```python
from build123d import *

# Parameters (mm, degrees)
SKETCH1_W           = 207.9625
SKETCH1_H           = 101.6
BOSS_EXTRUDE1_DEPTH = 6.35
SKETCH2_W           = 41.5925
SKETCH2_H           = 6.35
SKETCH2_W_2         = 35.2425
SKETCH2_W_3         = 6.35
SKETCH2_H_2         = 12.7
CUT_EXTRUDE1_DEPTH  = 6.35
SKETCH3_W           = 41.5925
SKETCH3_H           = 31.75
CUT_EXTRUDE2_DEPTH  = 6.35


with BuildPart() as part:
    # Sketch1 → Boss-Extrude1 (new body)
    with BuildSketch(Plane.XY):
        Rectangle(SKETCH1_W, SKETCH1_H)
    extrude(amount=BOSS_EXTRUDE1_DEPTH)

    # Sketch2 → Cut-Extrude1 (cut)
    with BuildSketch(Plane.XY.offset(6.35)):
        with Locations((0, 47.625)):
            Rectangle(SKETCH2_W, SKETCH2_H)
        with Locations((-83.185, 47.625)):
            Rectangle(SKETCH2_W, SKETCH2_H)
        with Locations((83.185, 47.625)):
            Rectangle(SKETCH2_W, SKETCH2_H)
        with Locations((80.01, -47.625)):
            Rectangle(SKETCH2_W_2, SKETCH2_H)
        with Locations((100.80625, -47.625)):
            Rectangle(SKETCH2_W_3, SKETCH2_H)
        with Locations((100.80625, -41.275)):
            Rectangle(SKETCH2_W_3, SKETCH2_H)
        with Locations((0, -47.625)):
            Rectangle(SKETCH2_W, SKETCH2_H)
        with Locations((-100.80625, -41.275)):
            Rectangle(SKETCH2_W_3, SKETCH2_H)
        with Locations((-100.80625, -47.625)):
            Rectangle(SKETCH2_W_3, SKETCH2_H)
        with Locations((-80.01, -47.625)):
            Rectangle(SKETCH2_W_2, SKETCH2_H)
        with Locations((-100.80625, 31.75)):
            Rectangle(SKETCH2_W_3, SKETCH2_H_2)
        with Locations((-100.80625, 6.35)):
            Rectangle(SKETCH2_W_3, SKETCH2_H_2)
        with Locations((-100.80625, -19.05)):
            Rectangle(SKETCH2_W_3, SKETCH2_H_2)
        with Locations((100.80625, -19.05)):
            Rectangle(SKETCH2_W_3, SKETCH2_H_2)
        with Locations((100.80625, 6.35)):
            Rectangle(SKETCH2_W_3, SKETCH2_H_2)
        with Locations((100.80625, 31.75)):
            Rectangle(SKETCH2_W_3, SKETCH2_H_2)
    extrude(amount=-CUT_EXTRUDE1_DEPTH, mode=Mode.SUBTRACT)

    # Sketch3 → Cut-Extrude2 (cut)
    with BuildSketch(Plane.XY.offset(6.35)):
        with Locations((83.185, 28.575)):
            Rectangle(SKETCH3_W, SKETCH3_H)
    extrude(amount=-CUT_EXTRUDE2_DEPTH, mode=Mode.SUBTRACT)


solid = part.part
```
Could you check a few things on this model? Use its own coordinates, in mm. A direction names the side the tool comes from. Give positions to 0.01 mm unless a question says otherwise; leave off trailing zeros. Order: outer loops, then holes, each group sorted by start corner. A loop starts at its lowest first (then second) coordinate and runs counter-clockwise, first axis right, second up.
Q1. If I drill on line 1 along X through (y, z) = (7.5, 6); line 2 along X through (y, z) = (35.5, 3); line 3 along Y through (x, z) = (-66, 2), over which ranges is the centre line in solid material (lowest first)?
Q2. For faces 1 (the flat face through (97.631, 6, 3)), 2 (the flat face through (101, -25.4, 3)), 3 (the flat face through (62.389, -48, 3)), 4 (the flat face through (-97.631, -41, 3)), 5 (the flat face through (-97.631, 32, 3)), which set-ups out of +Z, -Z, +X, -X, +Y, -Y let a thin tool reach every point of the face, with its end or its side?
Q3. I'm going to push flat-ended pins straight in: P1, Ø3, axis at y = -49, z = 3, coming from the -X side; P2, Ø3, axis at x = -100, z = 2, coming from the -Y side; P3, Ø1, axis at y = 10, z = 4, coming from the -X side. Where does each tip first touch, or does it pass through?
Q4. Suppose I cut it at B-B, the plane x = -73. Write out the boundary of the cut face in (y, z), and give its area (3 significant figures).
Q5. We'd pull the mould along Y, two halves only. Please class faces 6 (the flat face through (-101, -25.4, 3)), 7 (the flat face through (101, -38.1, 3)), 8 (the flat face through (20.796, -48, 3)): +Y half, -Y half, draft (parallel to the pull), parting line (faces both ways), or undercut.
Q6. Suppose I cut it at A-A, the plane y = -40. Write out the boundary of the cut face in (x, z).
Solution:
1. line 1: x = -97.63 to 97.63
1. line 2: x = -97.63 to 62.39
1. line 3: y = -44.45 to 44.45
2. face 1: +Z, -Z, +X, +Y
2. face 2: +Z, -Z, +X
2. face 3: +Z, -Z, +X, -Y
2. face 4: +Z, -Z, -X, -Y
2. face 5: +Z, -Z, -X
3. P1: stops at x = -62.39
3. P2: stops at y = -38.1
3. P3: stops at x = -97.63
4. outline: (-44.45, 0) - (44.45, 0) - (44.45, 6.35) - (-44.45, 6.35) - close
4. area: 565 mm2
5. face 6: undercut
5. face 7: -Y half
5. face 8: draft
6. outline: (-97.63, 0) - (97.63, 0) - (97.63, 6.35) - (-97.63, 6.35) - close
